Check sheet for the drawn part. Datum: minimum x, y, z corner. Units: mm. A direction names the side the tool comes from. Round coordinates to 2 decimals unless told otherwise and drop trailing zeros. Write each loop counter-clockwise with the first axis right and the second up, starting at its lowest first coordinate (ties: lowest second). Pieces come first, ordered by that corner, then holes. Notation, with made-up numbers: M 89,-23 L 132,-23 A11 cw 132,-15 Z; hole C 38.5,21 d9. An arc over 180 degrees is marked long. One line per item, written item: value. Start each with the question number.
Item 1: Section check A-A, the plane x = 12.7. Record the cut outline in (y, z) (1 decimal).
Item 2: Section check D-D, the plane y = 2. Record the cut outline in (x, z) (1 decimal), then the cut area to 3 significant figures.
Item 3: Tool access check on the marked faces 1 and 2. Record the directions out of +Z, -Z, +X, -X, +Y, -Y that give a thin tool (end or side, any length) a straight path to the whole face; none if there is none.
Item 4: Section check C-C, the plane z = 16.5. Record the cut outline in (x, y) (3 decimals), then the cut area to 3 significant figures.
Item 5: Thickness scan on probe 1 along X at (y, z) = (24.35, 12.7); probe 2 along Z at (x, y) = (43, 7.75) (3 decimals). Record the ranges inside material, lowest first. Write a range as from..to.
Item 6: Draft check along Z on the marked faces 3, 4 and 5. Enter one of: +Z half, -Z half, draft (parallel to the pull), parting line (faces both ways), or undercut.
Item 7: Section check B-B, the plane y = 12.7. Record the cut outline in (x, z) (1 decimal).
Item 8: Gauge pin test, flat end, axial feed: pin 1 (3 mm diameter, centred on y = 20.5, z = 5, fed in from -X). Record the tip position at first contact, or that the pin passes through.
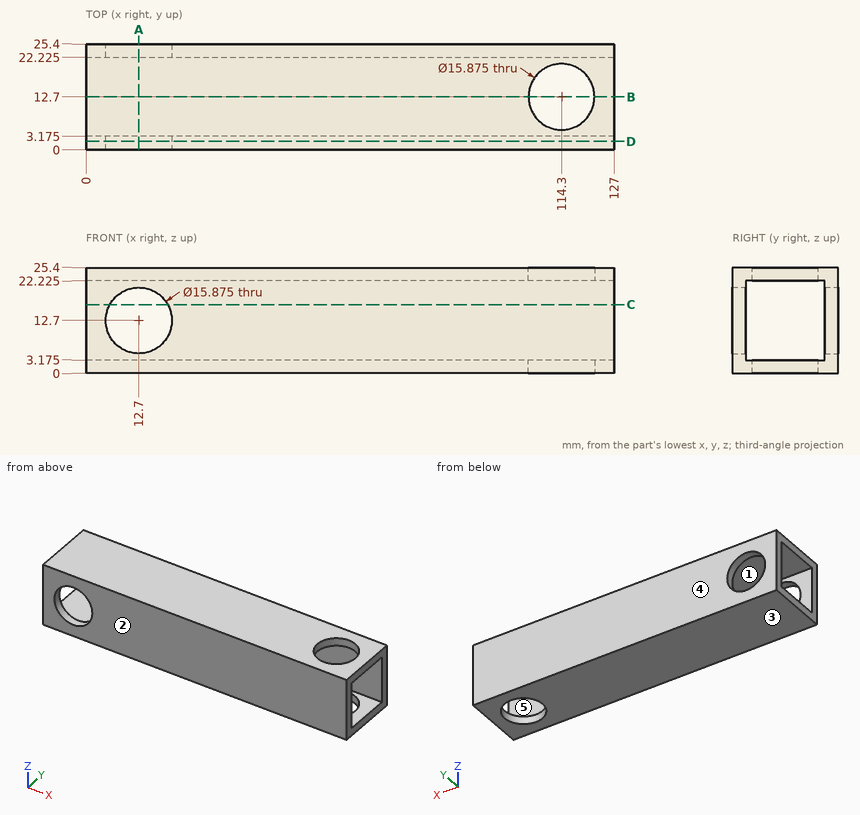
Response values:
1. outline: M 0,0 L 25.4,0 L 25.4,4.8 L 22.2,4.8 L 22.2,3.2 L 3.2,3.2 L 3.2,4.8 L 0,4.8 Z; M 0,20.6 L 3.2,20.6 L 3.2,22.2 L 22.2,22.2 L 22.2,20.6 L 25.4,20.6 L 25.4,25.4 L 0,25.4 Z
2. outline: M 0,0 L 127,0 L 127,25.4 L 0,25.4 Z; hole C 12.7,12.7 d15.9
2. area: 3,030 mm2
3. face 1: +X, -X
3. face 2: +Z, -Z, +X, -X, -Y
4. outline: M 0,0 L 5.731,0 L 5.731,3.175 L 0,3.175 Z; M 0,22.225 L 5.731,22.225 L 5.731,25.4 L 0,25.4 Z; M 19.669,0 L 127,0 L 127,3.175 L 19.669,3.175 Z; M 19.669,22.225 L 127,22.225 L 127,25.4 L 19.669,25.4 Z
4. area: 718 mm2
5. probe 1: x = 0..4.76, 20.64..127
5. probe 2: z = 0..3.175, 22.225..25.4
6. face 3: -Z half
6. face 4: draft
6. face 5: undercut
7. outline: M 0,0 L 106.4,0 L 106.4,3.2 L 0,3.2 Z; M 0,22.2 L 106.4,22.2 L 106.4,25.4 L 0,25.4 Z; M 122.2,0 L 127,0 L 127,3.2 L 122.2,3.2 Z; M 122.2,22.2 L 127,22.2 L 127,25.4 L 122.2,25.4 Z
8. pin 1: passes through
